Can you work these out from the drawing? Everything is in mm from the part's minimum corner. A direction names the side the tool comes from. Round coordinates to 2 decimals unless told otherwise and drop trailing zeros. Loops run counter-clockwise (first coordinate to the right, second up) from the corner with the lowest first, then second, coordinate; pieces in that order, holes last. Notation, with made-up numbers: M 75,41.25 L 80,41.25 A15 cw 80,61.25 Z; hole C 28.5,54 d10. An arc over 180 degrees is marked long. One line per question, with ' | ' between items. Start each with the question number.
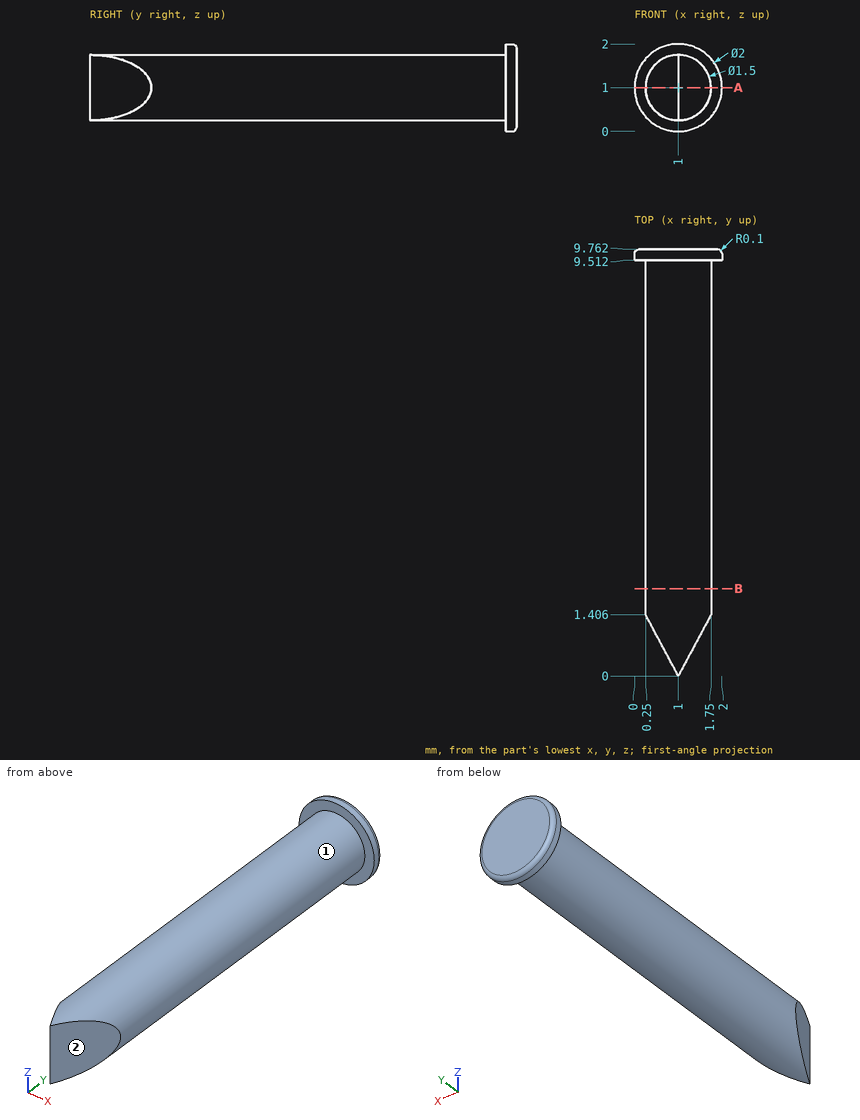
1) For the marked faces 1 and 2, which set-ups out of +Z, -Z, +X, -X, +Y, -Y let a thin tool reach every point of the face, with its end or its side?
2) Imagine slicing it at B-B (y = 2). Write out the boundary of the cut face in (x, z).
3) Please list where these lines run through material, in increasing order: L1, parallel to Y at x = 1.15, z = 1.8; L2, parallel to Y at x = 0.9, z = 0.75 (1 decimal); L3, parallel to X at y = 6, z = 0.55. Write a range as from..to.
4) Imagine slicing it at A-A (z = 1). Write out the boundary of the cut face in (x, y), then the cut area to 3 significant figures.
5) I'm going to push a flat-ended pin straight in: pin 1 Ø1 at (y, z) = (4, 1) entering from +X. Where does the tip first touch, or does it pass through?
Results are:
1) face 1: -Y | face 2: +Z, -Z, +X, -Y
2) outline: C 1,1 d1.5
3) L1: 9.51..9.76 | L2: 0.2..9.8 | L3: 0.4..1.6
4) outline: M 0,9.51 L 0.25,9.51 L 0.25,1.41 L 1,0 L 1.75,1.41 L 1.75,9.51 L 2,9.51 L 2,9.66 A0.1 ccw 1.9,9.76 L 0.1,9.76 A0.1 ccw 0,9.66 Z | area: 13.7 mm²
5) pin 1: x = 1.75
